Can you work these out from the model? Positions are in its coordinate system, mm. Face numbers are marked on the shaded views. A direction names the side the tool comes from. Round coordinates to 2 decimals unless told otherwise and drop trailing zeros. Order: outer loops, then holes, each group sorted by start corner. A loop starts at its lowest first (then second) coordinate and runs counter-clockwise, first axis right, second up.
Q1. If we section it at A-A (z = 7.5): Please give me the cut outline in (x, y) (3 decimals), plus the area to 3 significant figures.
Q2. We'd pull the mould along X, two halves only. Please class the marked faces 1, 2, 3 and 4: pulls with the +X half, pulls with the -X half, needs draft (parallel to the pull), parting line crosses it, or undercut.
Q3. If we section it at B-B (y = 37): Please give me the cut outline in (x, z) (3 decimals), plus the area to 3 significant figures.
Q4. Will these pins go through, and if not, where does the flat tip stop? P1, Ø10, axis at x = 41, z = 51.5, coming from the -Y side; P2, Ø10, axis at x = 82, z = 53, coming from the +Y side; P3, Ø3, axis at x = 86.5, y = -3, coming from the -Z side.
Q5. If I drill on line 1 (Z direction, x = -25.5, y = -39.5) (3 decimals); line 2 (Y direction, x = 21, z = 16); line 3 (Y direction, x = 37.5, z = 51.5), over which ranges is the centre line in solid material (lowest first)?
Q6. If we section it at C-C (x = 99.5): Please give me the cut outline in (y, z) (3 decimals).
Q7. For the marked faces 5, 6, 7 and 8, which set-ups out of +Z, -Z, +X, -X, +Y, -Y let a thin tool reach every point of the face, with its end or its side?
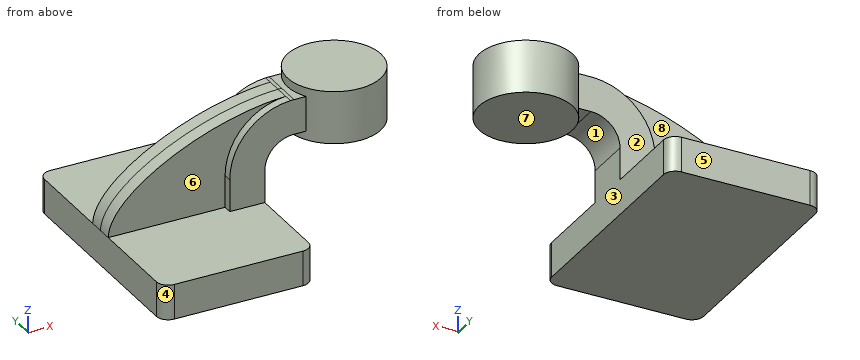
from build123d import *

# Parameters (mm, degrees)
F1_DEPTH = 63.5
F0_W     = 25.4
F0_H     = 19.05
F2_DEPTH = 12.7
F3_DEPTH = 7.9375
F5_R     = 6.35


with BuildPart() as f1:
    # F0 (on Front) → F1 (new body, symmetric)
    with BuildSketch(Plane.XZ):
        Polygon((22.225, 9.525), (-41.275, 9.525), (-41.275, -9.525), (41.275, -9.525), (41.275, 9.525), align=None)
    extrude(amount=F1_DEPTH, both=True)

    # F0 (on Front) → F2 (join, symmetric)
    with BuildSketch(Plane.XZ):
        with Locations((73.025, 52.4002)):
            Rectangle(F0_W, F0_H)
        with BuildLine():
            Line((22.225, 27.0002), (22.225, 9.525))
            Line((22.225, 9.525), (41.275, 9.525))
            Line((41.275, 9.525), (41.275, 27.0002))
            ThreePointArc((41.275, 27.0002), (45.9246798487, 38.2255201513), (57.15, 42.8752))
            Line((57.15, 42.8752), (60.325, 42.8752))
            Line((60.325, 42.8752), (60.325, 61.9252))
            Line((60.325, 61.9252), (57.15, 61.9252))
            add(Edge.make_bspline(
                [(55.2099659043, 61.8712753019), (55.8590535699, 61.8953003864), (56.5058041555, 61.9133112934), (57.15, 61.9252)],
                knots=[109.841532406, 109.841532406, 109.841532406, 109.841532406, 111.5045361635, 111.5045361635, 111.5045361635, 111.5045361635], degree=3))
            ThreePointArc((55.2099659043, 61.8712753019), (31.7776595897, 51.0001993147), (22.225, 27.0002))
        make_face()
    extrude(amount=F2_DEPTH, both=True)

    # F0 (on Front) → F3 (join, symmetric)
    with BuildSketch(Plane.XZ):
        with BuildLine():
            add(Edge.make_bspline(
                [(-41.275, 9.525), (-40.7303956796, 32.4600275426), (12.3376731995, 60.2844165268), (55.2099659043, 61.8712753019)],
                knots=[0, 0, 0, 0, 109.841532406, 109.841532406, 109.841532406, 109.841532406], degree=3))
            Line((-41.275, 9.525), (22.225, 9.525))
            Line((22.225, 9.525), (22.225, 27.0002))
            ThreePointArc((22.225, 27.0002), (31.7776595897, 51.0001993147), (55.2099659043, 61.8712753019))
        make_face()
    extrude(amount=F3_DEPTH, both=True)

    # F0 (on Front) → F4 (revolve)
    with BuildSketch(Plane.XZ):
        Polygon((85.725, 66.675), (85.725, 61.9252), (85.725, 42.8752), (85.725, 38.1), (111.125, 38.1), (111.125, 66.675), align=None)
    revolve(axis=Axis((85.725, 0, 52.3875), (0, 0, 1)))

    # F5
    f5_edges = [f1.edges().sort_by_distance(p)[0] for p in [
        (-41.275, -63.5, 0),
        (41.275, -63.5, 0),
        (41.275, 63.5, 0),
        (-41.275, 63.5, 0),
    ]]
    fillet(f5_edges, radius=F5_R)


solid = f1.part
Solution:
1. outline: (-41.275, -57.15) arc R6.35 ccw to (-34.925, -63.5) - (34.925, -63.5) arc R6.35 ccw to (41.275, -57.15) - (41.275, 57.15) arc R6.35 ccw to (34.925, 63.5) - (-34.925, 63.5) arc R6.35 ccw to (-41.275, 57.15) - close
1. area: 10,400 mm2
2. face 1: undercut
2. face 2: needs draft
2. face 3: pulls with the +X half
2. face 4: pulls with the -X half
3. outline: (-41.275, -9.525) - (41.275, -9.525) - (41.275, 9.525) - (-41.275, 9.525) - close
3. area: 1,570 mm2
4. P1: stops at y = -12.7
4. P2: stops at y = 25.4
4. P3: stops at z = 38.1
5. line 1: z = -9.525 to 9.525
5. line 2: y = -7.94 to 7.94
5. line 3: y = -12.7 to 12.7
6. outline: (-21.34, 38.1) - (21.34, 38.1) - (21.34, 66.675) - (-21.34, 66.675) - close
7. face 5: +Z, -Z, +X, -X, +Y
7. face 6: +Z, -X, -Y
7. face 7: -Z, +X, +Y, -Y
7. face 8: +Z, -X, +Y
